Geometry: final body of the model. Coordinates: model frame, mm. Round coordinates to 2 decimals unless told otherwise and drop trailing zeros. Loops run counter-clockwise (first coordinate to the right, second up) from the corner with the lowest first, then second, coordinate; pieces in that order, holes last. Notation, with made-up numbers: M 78.25,17 L 116.25,17 A24 cw 116.25,39 Z; hole C -25,-3.75 d3. An arc over 180 degrees is marked long. Answer as a JSON object with one key per item and string values.
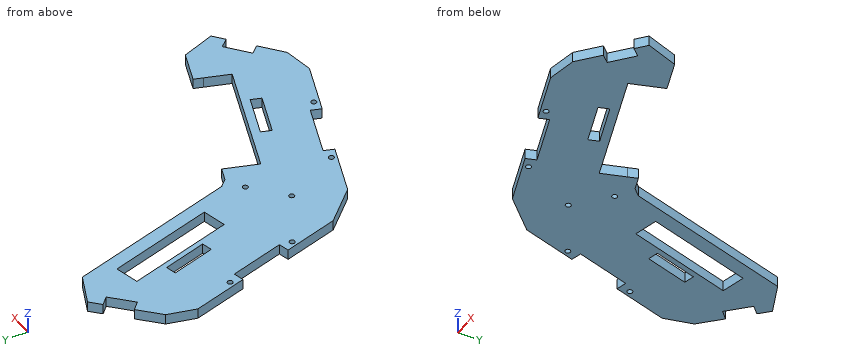
```python
from build123d import *

# Parameters (mm, degrees)
SALIENTE_EXTRUIR1_DEPTH = 5
CROQUIS2_R              = 1.25
CORTAR_EXTRUIR1_DEPTH   = 10
CORTAR_EXTRUIR2_DEPTH   = 10
CORTAR_EXTRUIR3_DEPTH   = 10
CORTAR_EXTRUIR4_DEPTH   = 22
CORTAR_EXTRUIR5_DEPTH   = 10
SALIENTE_EXTRUIR3_DEPTH = 5
CORTAR_EXTRUIR7_DEPTH   = 5
CROQUIS9_R              = 1.25
CORTAR_EXTRUIR6_DEPTH   = 10


with BuildPart() as part:
    # Croquis1 → Saliente-Extruir1 (new body)
    with BuildSketch(Plane.XY):
        Polygon((94.71302301, -28.670259317), (124.784571975, -2.294096918), (121.487551675, 1.464846702), (33.971255169, 31.023525729), (29.162783478, 36.110627065), (4.554636507, 125.156882092), (0.987169784, 128.660192123), (-27.039310471, 100.120458339), (-30.489528096, 86.717422014), (-9.088639631, 9.652046375), (5.402210696, -5.678484568), (81.141270829, -31.381887447), align=None)
    extrude(amount=SALIENTE_EXTRUIR1_DEPTH)

    # Croquis2 → Cortar-Extruir1 (cut)
    with BuildSketch(Plane.XY.offset(5)):
        with Locations((27.933375513, 30.132453761)):
            Circle(CROQUIS2_R)
        with Locations((13.398800269, 16.393963215)):
            Circle(CROQUIS2_R)
    extrude(amount=-CORTAR_EXTRUIR1_DEPTH, mode=Mode.SUBTRACT)

    # Croquis3 → Cortar-Extruir2 (cut)
    with BuildSketch(Plane(origin=(0, 0, 0), x_dir=(-1, 0, 0), z_dir=(0, 0, -1))):
        Polygon((-93.962142428, -1.904403336), (-37.71071672, 17.094547759), (-41.550617787, 28.463591685), (-97.802043495, 9.46464059), align=None)
    extrude(amount=-CORTAR_EXTRUIR2_DEPTH, mode=Mode.SUBTRACT)

    # Croquis4 → Cortar-Extruir3 (cut)
    with BuildSketch(Plane(origin=(0, 0, 0), x_dir=(-1, 0, 0), z_dir=(0, 0, -1))):
        Polygon((-11.35589305, 49.864341228), (2.384432549, 99.58464479), (-8.700088084, 102.647878755), (-22.440413684, 52.927575193), align=None)
    extrude(amount=-CORTAR_EXTRUIR3_DEPTH, mode=Mode.SUBTRACT)

    # Croquis5 → Cortar-Extruir4 (cut)
    with BuildSketch(Plane(origin=(0, 0, 0), x_dir=(-1, 0, 0), z_dir=(0, 0, -1))):
        Polygon((23.359165427, 61.040727405), (18.541476581, 62.378589198), (11.406213682, 36.684248684), (16.223902529, 35.34638689), align=None)
        Polygon((-55.889136713, -22.812124691), (-57.49596723, -18.077349544), (-32.243833114, -9.507586787), (-30.637002597, -14.242361934), align=None)
        Polygon((-101.439852365, -16.119261564), (-111.46370202, -7.327207431), (-114.76072232, -11.086151051), (-104.736872665, -19.878205184), align=None)
        Polygon((14.129683663, 106.130392902), (4.787523578, 115.643637497), (8.354990301, 119.146947529), (17.697150386, 109.633702934), align=None)
    extrude(amount=-CORTAR_EXTRUIR4_DEPTH, mode=Mode.SUBTRACT)

    # Croquis6 → Cortar-Extruir5 (cut)
    with BuildSketch(Plane(origin=(0, 0, 0), x_dir=(-1, 0, 0), z_dir=(0, 0, -1))):
        Polygon((-55.751519014, 6.80303632), (-75.953226307, -0.052773886), (-74.34639579, -4.787549032), (-54.144688498, 2.068261173), align=None)
        Polygon((0.798726555, 84.444359548), (-4.909483764, 63.888887136), (-0.091794917, 62.551025343), (5.616415401, 83.106497755), align=None)
    extrude(amount=-CORTAR_EXTRUIR5_DEPTH, mode=Mode.SUBTRACT)

    # Croquis10 → Saliente-Extruir3 (add)
    with BuildSketch(Plane(origin=(0, 0, 0), x_dir=(-1, 0, 0), z_dir=(0, 0, -1))):
        Polygon((-121.487551675, 1.464846702), (-97.802043495, 9.46464059), (-99.242006394, 13.728032063), (-122.927514575, 5.728238174), align=None)
        Polygon((-29.162783478, 36.110627065), (-4.554636507, 125.156882092), (-8.892057625, 126.355538861), (-33.202024845, 38.388267562), (-36.472242051, 34.928555747), (-42.990580687, 32.726983158), (-41.550617787, 28.463591685), (-33.971255169, 31.023525729), align=None)
    extrude(amount=-SALIENTE_EXTRUIR3_DEPTH)

    # Croquis11 → Cortar-Extruir7 (cut)
    with BuildSketch(Plane(origin=(0, 0, 0), x_dir=(-1, 0, 0), z_dir=(0, 0, -1))):
        Polygon((-119.772647147, -6.690123985), (-114.40073163, 8.608163974), (-122.927514575, 5.728238174), (-121.487551675, 1.464846702), (-124.784571975, -2.294096918), align=None)
        Polygon((3.683910258, 123.903569826), (-11.289371163, 117.680696626), (-8.892057625, 126.355538861), (-4.554636507, 125.156882092), (-0.987169784, 128.660192123), align=None)
    extrude(amount=-CORTAR_EXTRUIR7_DEPTH, mode=Mode.SUBTRACT)

    # Croquis9 → Cortar-Extruir6 (cut)
    with BuildSketch(Plane(origin=(0, 0, 0), x_dir=(-1, 0, 0), z_dir=(0, 0, -1))):
        with Locations((-26.705642709, -10.268143844)):
            Circle(CROQUIS9_R)
        with Locations((-61.427327118, -22.051567634)):
            Circle(CROQUIS9_R)
        with Locations((12.477196312, 31.19762894)):
            Circle(CROQUIS9_R)
        with Locations((22.288182797, 66.527347148)):
            Circle(CROQUIS9_R)
    extrude(amount=-CORTAR_EXTRUIR6_DEPTH, mode=Mode.SUBTRACT)


solid = part.part
```
1) First-contact query: pin 1 (2 mm diameter, centred on x = -22.29, y = 66.53, fed in from -Z); pin 2 (3 mm diameter, centred on y = 100.5, z = 2, fed in from -X). Flat tips, straight axial feed; report the tip coordinate or a pass-through.
Geometry results:
{"pin 1": "through", "pin 2": "x = -27.33"}
2) Cut plane B-B on y = 96. Return the cut outline in (x, z).
Geometry results:
{"outline": "M -28.1,0 L -1.39,0 L -1.39,5 L -28.1,5 Z; M 10.54,0 L 17.28,0 L 17.28,5 L 10.54,5 Z"}
3) Cut plane C-C on z = 3.4. Count the separate pieces of the cut face and the enclosed holes in it, and give its area (3 significant figures).
Geometry results:
{"separate pieces": "1", "enclosed holes": "9", "area": "7,260 mm2"}
4) Cut plane D-D on x = 49.5. Return the cut outline in (y, z).
Geometry results:
{"outline": "M -15.36,0 L 13.11,0 L 13.11,5 L -15.36,5 Z"}
5) Line query: probe 1 along Y at (x, z) = (62, 2.65); probe 2 along X at (y, z) = (82, 2.8); probe 3 along X at (y, z) = (64.5, 0.8). Output: solid intervals per line, ascending.
Geometry results:
{"probe 1": "-24.89 to -23.16, -20.94 to -0.6, 4.68 to 8.89", "probe 2": "-29.18 to -5.31, -0.12 to 2.48, 14.41 to 21.15", "probe 3": "-24.32 to -0.45, 4.74 to 7.31, 19.24 to 25.99"}
6) Cut plane A-A on y = 71. Return the cut outline in (x, z) (3 decimals).
Geometry results:
{"outline": "M -26.125,0 L -2.254,0 L -2.254,5 L -26.125,5 Z; M 2.935,0 L 5.515,0 L 5.515,5 L 2.935,5 Z; M 17.446,0 L 24.19,0 L 24.19,5 L 17.446,5 Z"}
